For this review, use the dimensioned drawing (mm, ordinates from the lowest corner) and the shaded views. A direction names the side the tool comes from. Coordinates: 2 decimals unless noted, no trailing zeros. Loops run counter-clockwise (first coordinate to the right, second up) from the corner with the lowest first, then second, coordinate; pieces in that order, holes last. Notation, with made-up numbers: M 41.25,56.25 L 69.25,56.25 A19 ccw 69.25,76.25 Z; hole C 35,71.5 d4. An arc over 180 degrees is marked long. Write item = value, one per line. Start each with the question number.
Q1. For the marked faces 5 and 6, list the 3-axis set-ups (+Z, -Z, +X, -X, +Y, -Y) from which the entire face can be reached by the end or side of a thin tool; tool diameter is ignored.
Q2. Clearance check with flat-ended pins moving along their axes: pin 1 Ø2 at (x, z) = (9, 65) entering from -Y; pin 2 Ø2 at (y, z) = (51, 25.5) entering from -X. State where each tip first meets the part, or that it passes through.
Q3. We need section B-B on x = 3.25. Give the boundary of the cut face in (y, z), and give its area (3 significant figures).
Q4. We need section D-D on y = 53. Give the boundary of the cut face in (x, z).
Q5. We need section A-A on y = 6.5. Give the boundary of the cut face in (x, z), and give its area (3 significant figures).
Q6. Wall thickness on probe 1 along Z at (x, y) = (13.5, 25.5); probe 2 along Y at (x, z) = (16.75, 28.5); probe 3 along X at (y, z) = (23, 68): over which ranges is each line inside the solid? List them lowest first.
Q7. We need section C-C on z = 9. Give the boundary of the cut face in (x, y), and give its area (3 significant figures).
Q8. Mouldability with a two-part tool opening along Z and no side actions: class the marked faces 1, 2, 3 and 4 as released by +Z, released by -Z, zero draft, split by the parting line, or undercut.
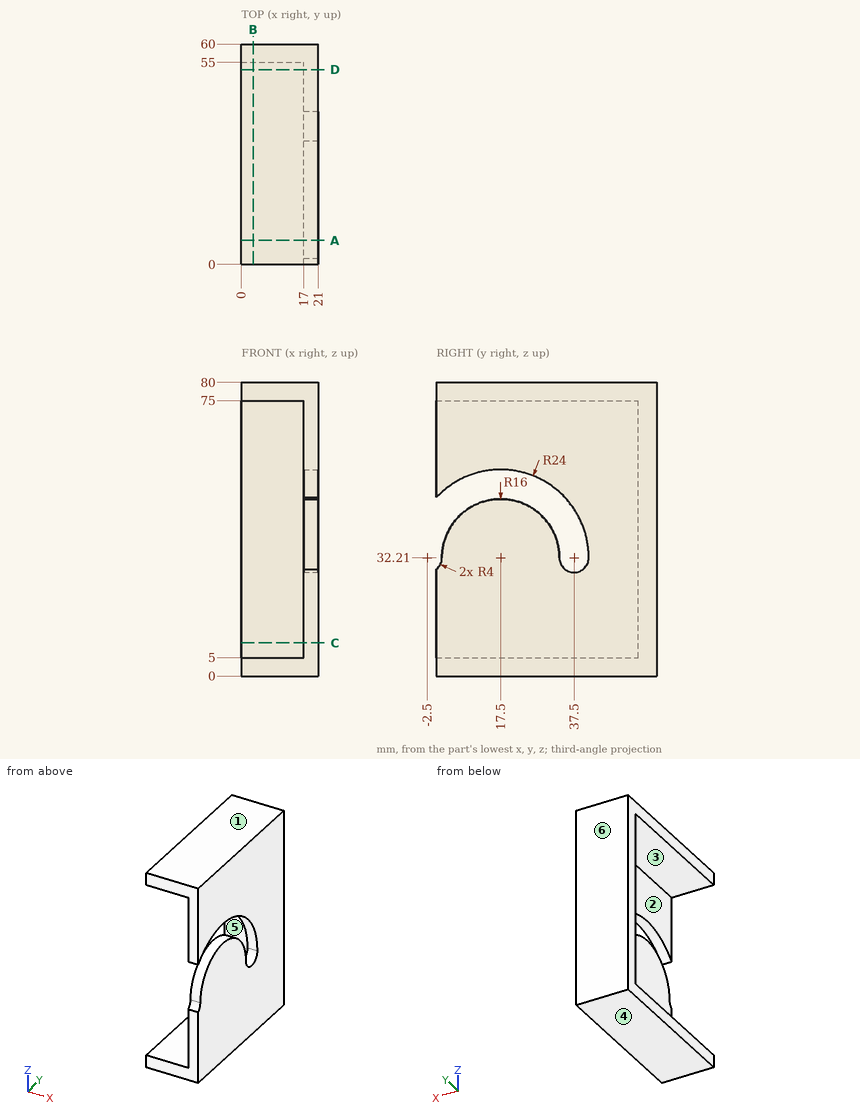
Returned:
q1.face_5 = -X, -Y
q1.face_6 = +Z, -Z, +X, -X, +Y
q2.pin_1 = 55
q2.pin_2 = 17
q3.outline = M 0,0 L 60,0 L 60,80 L 0,80 L 0,75 L 55,75 L 55,5 L 0,5 Z
q3.area = 950 mm^2
q4.outline = M 0,0 L 21,0 L 21,80 L 0,80 L 0,75 L 17,75 L 17,5 L 0,5 Z
q5.outline = M 0,0 L 21,0 L 21,43.83 L 17,43.83 L 17,5 L 0,5 Z; M 0,75 L 17,75 L 17,53.54 L 21,53.54 L 21,80 L 0,80 Z
q5.area = 451 mm^2
q6.probe_1 = 0 to 5, 75 to 80
q6.probe_2 = 55 to 60
q6.probe_3 = 17 to 21
q7.outline = M 0,55 L 17,55 L 17,0 L 21,0 L 21,60 L 0,60 Z
q7.area = 325 mm^2
q8.face_1 = released by +Z
q8.face_2 = undercut
q8.face_3 = undercut
q8.face_4 = released by -Z
